Autodesk Inventor part; units mm, degrees
ref_plane "YZ Plane" through (0, 0, 0) normal (1, 0, 0) x (0, 1, 0)
ref_plane "XZ Plane" through (0, 0, 0) normal (0, 1, 0) x (-1, 0, 0)
ref_plane "XY Plane" through (0, 0, 0) normal (0, 0, 1) x (1, 0, 0)
sketch "Sketch1" plane through (0, 0, 0) normal (0, 1, 0) x (-1, 0, 0)
  line L0 (12.6229, 24.94) -> (0, 24.94)
  line L1 (0, 24.94) -> (0, -8.3425)
  line L2 (0, -8.3425) -> (12.6229, -8.3425)
  line L3 (12.6229, -8.3425) -> (12.6229, 24.94)
  line L4 (12.6229, 24.94) -> (0, -8.3425) construction
  line L5 (0, 24.94) -> (12.6229, -8.3425) construction
  point P0 (0, 0)
  point P1 (6.3114, 8.2988)
extrude "Extrusion1" add sketch "Sketch1" along normal blind 10
sketch "Sketch2" plane through (0, 10, 0) normal (0, 1, 0) x (1, 0, 0)
  circle A0 centre (-6.1347, -9.4794) radius 5.954
  point P0 (0, 0)
extrude "Extrusion2" add sketch "Sketch2" along normal blind 10
properties part number "mass applied" material "Iron, Cast"
Geometry check sheet. Reference: the model listing, model coordinates, mm. A direction names the side the tool comes from. Give positions to 0.01 mm unless a question says otherwise; leave off trailing zeros. Loops run counter-clockwise (first coordinate to the right, second up) from the corner with the lowest first, then second, coordinate; pieces in that order, holes last. Notation, with made-up numbers: (68, 31.5) -> (101, 31.5) arc R11 cw to (101, 49.5) -> close; hole circle Ø2 at (50.25, -22). An arc over 180 degrees is marked (long way). Answer in a Markdown table with one row per item. Add a question column.
1) Set-up check for faces 1 (the face through (-3.387, 14.93, 4.197)), 2 (the face through (-6, 20, 9)): record each of +Z, -Z, +X, -X, +Y, -Y from which the full face is reachable in a straight line by a thin tool's end or side.
2) Cross-section at B-B on x = -10.5. Record the boundary of the cut face in (y, z).
3) Cross-section at A-A on z = 5. Record the boundary of the cut face in (x, y).
4) Material ranges on probe 1 along Y at (x, z) = (-1, 2); probe 2 along Z at (x, y) = (-4, 19); probe 3 along X at (y, z) = (14.5, 4.5), recorded low to high. Write a range as from..to.
5) Cross-section at C-C on z = 19.5. Record the boundary of the cut face in (x, y).
6) Cross-section at D-D on y = 18.25. Record the boundary of the cut face in (x, z), and give its area (3 significant figures).
7) Gauge pin test, flat ends, axial feed: P1, Ø4, axis at y = 17, z = 15.5, coming from the -X side; P2, Ø8, axis at y = 15, z = 2, coming from the +X side; P3, Ø3, axis at y = 14, z = 1.5, coming from the -X side; P4, Ø4, axis at x = -10, z = 3, coming from the +Y side. Record the tip position at first contact, or that the pin passes through.
Outcome:
| question | item | result |
|---|---|---|
| 1 | face 1 | +Y |
| 1 | face 2 | +Z, -Z, +X, -X, +Y |
| 2 | outline | (0, -8.34) -> (10, -8.34) -> (10, 5.43) -> (20, 5.43) -> (20, 13.53) -> (10, 13.53) -> (10, 24.94) -> (0, 24.94) -> close |
| 3 | outline | (-12.62, 0) -> (0, 0) -> (0, 10) -> (-2.21, 10) -> (-2.21, 20) -> (-10.06, 20) -> (-10.06, 10) -> (-12.62, 10) -> close |
| 4 | probe 1 | y = 0..10 |
| 4 | probe 2 | z = 3.92..15.04 |
| 4 | probe 3 | x = -9.4..-2.87 |
| 5 | outline | (-12.62, 0) -> (0, 0) -> (0, 10) -> (-12.62, 10) -> close |
| 6 | outline | circle Ø11.91 at (-6.13, 9.48) |
| 6 | area | 111 mm^2 |
| 7 | P1 | stops at x = -10.53 |
| 7 | P2 | stops at x = -1.3 |
| 7 | P3 | passes through |
| 7 | P4 | stops at y = 20 |
